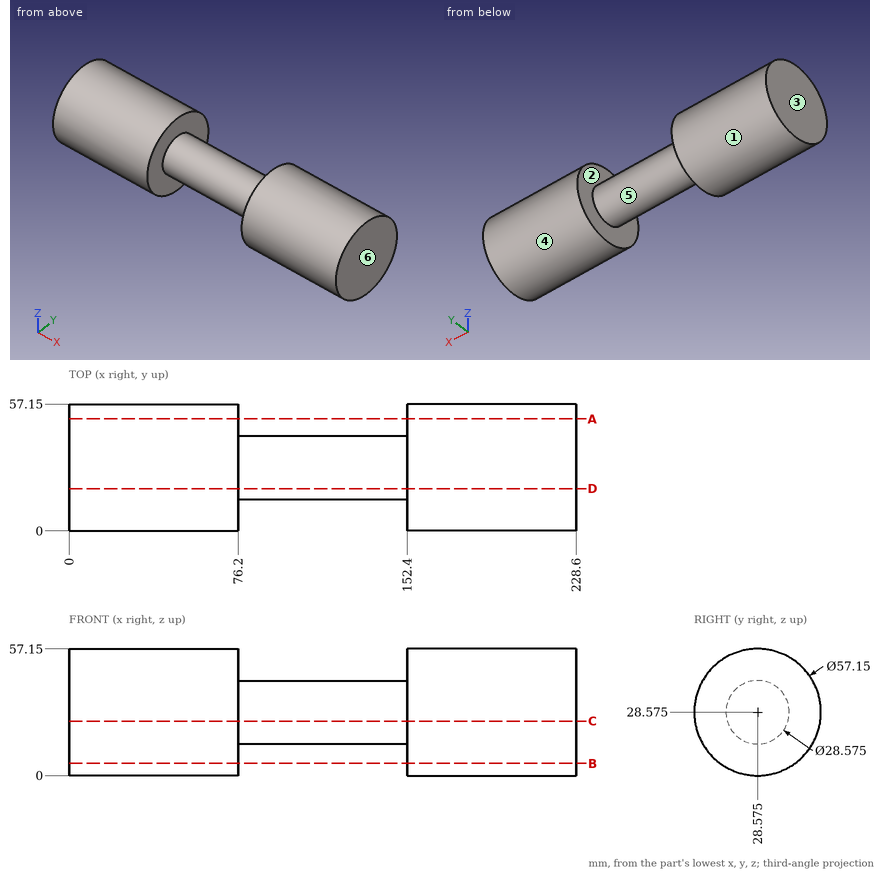
For this review, use the dimensioned drawing (mm, ordinates from the lowest corner) and the shaded views. A direction names the side the tool comes from. Give positions to 0.01 mm unless a question says otherwise; leave off trailing zeros. Order: outer loops, then holes, each group sorted by start corner. A loop starts at its lowest first (then second) coordinate and runs counter-clockwise, first axis right, second up. Notation, with made-up numbers: (70.5, -19) - (75.5, -19) arc R19 cw to (75.5, -9) - close; hole circle Ø8 at (69.25, 29). An arc over 180 degrees is marked (long way). Write item = value, one per line. Start each with the question number.
Q1. We need section A-A on y = 50.5. State the section outline as (x, z) points, plus the area to 3 significant figures.
Q2. We need section C-C on z = 24.5. State the section outline as (x, y) points, plus the area to 3 significant figures.
Q3. Mouldability with a two-part tool opening along X and no side actions: class the marked faces 3, 4, 5 and 6 as released by +X, released by -X, zero draft, split by the parting line, or undercut.
Q4. Tool access review of the marked faces 1 and 2: name each direction out of +Z, -Z, +X, -X, +Y, -Y from which nothing blocks a thin tool from reaching the whole face with its end or side.
Q5. We need section B-B on z = 5.5. State the section outline as (x, y) points, plus the area to 3 significant figures.
Q6. We need section D-D on y = 19. State the section outline as (x, z) points, plus the area to 3 significant figures.
Q7. Clearance check with flat-ended pins moving along their axes: pin 1 Ø5 at (x, z) = (71, 23) entering from +Y; pin 2 Ø10 at (x, y) = (136.5, 51) entering from +Z; pin 3 Ø6 at (x, z) = (86.5, 40.5) entering from +Y; pin 4 Ø1 at (x, y) = (29.5, 37.5) entering from +Z. State where each tip first meets the part, or that it passes through.
Q8. To check wall thickness, follow L1, parallel to X at y = 45.5, z = 34.5; L2, parallel to Y at x = 134, z = 41.5; L3, parallel to Y at x = 75, z = 20.5. State the ranges of each line that lie inside material, in increasing order. Write a range as from..to.
Working result:
q1.outline = (0, 10.25) - (76.2, 10.25) - (76.2, 46.9) - (0, 46.9) - close; (152.4, 10.25) - (228.6, 10.25) - (228.6, 46.9) - (152.4, 46.9) - close
q1.area = 5,590 mm²
q2.outline = (0, 0.29) - (76.2, 0.29) - (76.2, 14.88) - (152.4, 14.88) - (152.4, 0.29) - (228.6, 0.29) - (228.6, 56.86) - (152.4, 56.86) - (152.4, 42.27) - (76.2, 42.27) - (76.2, 56.86) - (0, 56.86) - close
q2.area = 10,700 mm²
q3.face_3 = released by -X
q3.face_4 = zero draft
q3.face_5 = undercut
q3.face_6 = released by +X
q4.face_1 = +X, -X
q4.face_2 = none
q5.outline = (0, 11.72) - (76.2, 11.72) - (76.2, 45.43) - (0, 45.43) - close; (152.4, 11.72) - (228.6, 11.72) - (228.6, 45.43) - (152.4, 45.43) - close
q5.area = 5,140 mm²
q6.outline = (0, 1.65) - (76.2, 1.65) - (76.2, 17.97) - (152.4, 17.97) - (152.4, 1.65) - (228.6, 1.65) - (228.6, 55.5) - (152.4, 55.5) - (152.4, 39.18) - (76.2, 39.18) - (76.2, 55.5) - (0, 55.5) - close
q6.area = 9,820 mm²
q7.pin_1 = 56.98
q7.pin_2 = through
q7.pin_3 = 39.73
q7.pin_4 = 55.88
q8.L1 = 0..76.2, 152.4..228.6
q8.L2 = 22.49..34.66
q8.L3 = 1.16..55.99
